Here's how the part is built. I have some questions about the finished solid (model axes, mm). A direction names the side the tool comes from. Round coordinates to 2 decimals unless told otherwise and drop trailing zeros. Order: outer loops, then holes, each group sorted by start corner. A loop starts at its lowest first (then second) coordinate and runs counter-clockwise, first axis right, second up. Notation, with made-up numbers: M 24.25,-4.75 L 34.25,-4.75 A28 ccw 34.25,24.25 Z; hole C -32.75,43.5 d7. An arc over 180 degrees is marked long. Write each question's results on one line, items separated by ' | '. Start each with the question number.
```python
from build123d import *

# Parameters (mm, degrees)
BOSS_EXTRUDE1_DEPTH = 60
CUT_EXTRUDE1_DEPTH  = 60
CHAMFER1_SIZE       = 1


with BuildPart() as part:
    # Sketch1 → Boss-Extrude1 (new body)
    with BuildSketch(Plane.XY):
        Polygon((-13.372093023, -14.244186047), (-7.598590331, -24.244186047), (16.627906977, -24.244186047), (16.627906977, -22.744186047), (-6.732564928, -22.744186047), (-11.872093023, -13.842262258), (-11.872093023, 15.755813953), (-13.372093023, 15.755813953), align=None)
    extrude(amount=BOSS_EXTRUDE1_DEPTH)

    # Sketch3 → Cut-Extrude1 (cut)
    with BuildSketch(Plane.ZY.offset(13.372093023)):
        with BuildLine():
            Line((8.25, 11.755813953), (8.25, 7.755813953))
            ThreePointArc((8.25, 7.755813953), (10, 6.005813953), (11.75, 7.755813953))
            Line((11.75, 7.755813953), (11.75, 11.755813953))
            ThreePointArc((11.75, 11.755813953), (10, 13.505813953), (8.25, 11.755813953))
        make_face()
        with BuildLine():
            Line((48.25, 11.755813953), (48.25, 7.755813953))
            ThreePointArc((48.25, 7.755813953), (50, 6.005813953), (51.75, 7.755813953))
            Line((51.75, 7.755813953), (51.75, 11.755813953))
            ThreePointArc((51.75, 11.755813953), (50, 13.505813953), (48.25, 11.755813953))
        make_face()
    extrude(amount=-CUT_EXTRUDE1_DEPTH, mode=Mode.SUBTRACT)

    # Chamfer1
    chamfer1_edges = [part.edges().sort_by_distance(p)[0] for p in [
        (16.627906977, -23.494186047, 60),
        (-12.622093023, 15.755813953, 60),
        (-12.622093023, 15.755813953, 0),
        (16.627906977, -23.494186047, 0),
    ]]
    chamfer(chamfer1_edges, length=CHAMFER1_SIZE)


solid = part.part
```
(1) I want a section at C-C on y = -9.5. Write out the boundary of the cut face in (x, z), and give its area (3 significant figures).
(2) Please list where these lines run through material, in increasing order: line 1 (X direction, y = -12, z = 3.5); line 2 (Y direction, x = 9, z = 52.5); line 3 (Y direction, x = -7.75, z = 25.5).
(3) I want a section at A-A on z = 10. Write out the boundary of the cut face in (x, y).
(4) If we mould it in two halves opening along Z, with no side actions, what happens to faces 1 (the cylindrical face through (-12.633, 13.505, 50.038)), 2 (the flat face through (-10, -18, 0)), 3 (the flat face through (-10, -18, 60))? For each: pulls with the +Z half, pulls with the -Z half, needs draft (parallel to the pull), parting line crosses it, or undercut.
(5) On a 3-axis mill with a long thin cutter (end or side, diameter ignored), from which of +Z, -Z, +X, -X, +Y, -Y can I reach the whole of each face in a straight line? I mean faces 4 (the flat face through (16.628, -24, 30)), 5 (the flat face through (-13, 10, 8.25)), 6 (the flat face through (5, -22.744, 30)). Say none if no direction works.
(6) I'm going to push flat-ended pins straight in: pin 1 Ø3 at (x, z) = (-9.5, 16.5) entering from -Y; pin 2 Ø8 at (x, z) = (2, 9) entering from +Y; pin 3 Ø1 at (x, z) = (-10, 22.5) entering from -Y. Where does each tip first touch, or does it pass through?
(7) I want a section at B-B on x = 9. Write out the boundary of the cut face in (y, z), and give its area (3 significant figures).
Solutions:
1) outline: M -13.37,0 L -11.87,0 L -11.87,60 L -13.37,60 Z | area: 90.0 mm^2
2) line 1: -13.37 to -11.87 | line 2: -24.24 to -22.74 | line 3: -23.98 to -20.98
3) outline: M -13.37,-14.24 L -7.6,-24.24 L 16.63,-24.24 L 16.63,-22.74 L -6.73,-22.74 L -11.87,-13.84 L -11.87,6.01 L -13.37,6.01 Z; M -13.37,13.51 L -11.87,13.51 L -11.87,15.76 L -13.37,15.76 Z
4) face 1: undercut | face 2: pulls with the -Z half | face 3: pulls with the +Z half
5) face 4: +Z, -Z, +X, +Y, -Y | face 5: +X, -X | face 6: +Z, -Z, +X, +Y
6) pin 1: y = -23.55 | pin 2: y = -22.74 | pin 3: y = -20.95
7) outline: M -24.24,0 L -22.74,0 L -22.74,60 L -24.24,60 Z | area: 90.0 mm^2
